Could you check a few things on this model? Use its own coordinates, in mm. A direction names the side the tool comes from. Round coordinates to 2 decimals unless told otherwise and drop trailing zeros. Order: outer loops, then holes, each group sorted by start corner. A loop starts at its lowest first (then second) coordinate and runs counter-clockwise, first axis right, second up.
```python
from build123d import *

# Parameters (mm, degrees)
SKETCH1_W           = 190
SKETCH1_H           = 80
SKETCH1_R           = 1.55
BOSS_EXTRUDE1_DEPTH = 2
SKETCH2_R           = 3
SKETCH2_R_2         = 1.55
BOSS_EXTRUDE2_DEPTH = 12


with BuildPart() as part:
    # Sketch1 → Boss-Extrude1 (new body)
    with BuildSketch(Plane(origin=(0, 0, 0), x_dir=(1, 0, 0), z_dir=(0, 1, 0))):
        with Locations((19.251207729, 0.579710145)):
            Rectangle(SKETCH1_W, SKETCH1_H)
        with Locations(Location((-72.748792271, 37.579710145, 0), (0, 0, 270))):
            Circle(SKETCH1_R, mode=Mode.SUBTRACT)
        with Locations(Location((111.435917928, 37.579710145, 0), (0, 0, 270))):
            Circle(SKETCH1_R, mode=Mode.SUBTRACT)
        with Locations(Location((111.435917928, -36.420289855, 0), (0, 0, 270))):
            Circle(SKETCH1_R, mode=Mode.SUBTRACT)
        with Locations(Location((-72.748792271, -36.420289855, 0), (0, 0, 270))):
            Circle(SKETCH1_R, mode=Mode.SUBTRACT)
    extrude(amount=BOSS_EXTRUDE1_DEPTH)

    # Sketch2 → Boss-Extrude2 (add)
    # profile 1 of 5: a face of its own
    with BuildSketch(Plane(origin=(0, 2, 0), x_dir=(1, 0, 0), z_dir=(0, 1, 0))):
        with Locations(Location((82.711207729, 24.709710145, 0), (0, 0, 270))):
            Circle(SKETCH2_R)
        with Locations(Location((82.711207729, 24.709710145, 0), (0, 0, 270))):
            Circle(SKETCH2_R_2, mode=Mode.SUBTRACT)
    # profile 2 of 5: a face of its own
    with BuildSketch(Plane(origin=(0, 2, 0), x_dir=(1, 0, 0), z_dir=(0, 1, 0))):
        with Locations(Location((80.711207729, -23.550289855, 0), (0, 0, 270))):
            Circle(SKETCH2_R)
        with Locations(Location((80.711207729, -23.550289855, 0), (0, 0, 270))):
            Circle(SKETCH2_R_2, mode=Mode.SUBTRACT)
    # profile 3 of 5: a face of its own
    with BuildSketch(Plane(origin=(0, 2, 0), x_dir=(1, 0, 0), z_dir=(0, 1, 0))):
        with Locations(Location((30.141207729, -8.310289855, 0), (0, 0, 270))):
            Circle(SKETCH2_R)
        with Locations(Location((30.141207729, -8.310289855, 0), (0, 0, 270))):
            Circle(SKETCH2_R_2, mode=Mode.SUBTRACT)
    # profile 4 of 5: a face of its own
    with BuildSketch(Plane(origin=(0, 2, 0), x_dir=(1, 0, 0), z_dir=(0, 1, 0))):
        with Locations(Location((-67.258792271, 33.649710145, 0), (0, 0, 270))):
            Circle(SKETCH2_R)
        with Locations(Location((-67.258792271, 33.649710145, 0), (0, 0, 270))):
            Circle(SKETCH2_R_2, mode=Mode.SUBTRACT)
    # profile 5 of 5: a face of its own
    with BuildSketch(Plane(origin=(0, 2, 0), x_dir=(1, 0, 0), z_dir=(0, 1, 0))):
        with Locations(Location((-67.748792271, -31.930289855, 0), (0, 0, 270))):
            Circle(SKETCH2_R)
        with Locations(Location((-67.748792271, -31.930289855, 0), (0, 0, 270))):
            Circle(SKETCH2_R_2, mode=Mode.SUBTRACT)
    extrude(amount=BOSS_EXTRUDE2_DEPTH)


solid = part.part
```
Q1. Imagine slicing it at B-B, the plane x = 50.5. Please give me the cut outline in (y, z), then the cut area to 3 significant figures.
Q2. For P1, Ø2.5, axis at x = -67.26, z = -33.65, coming from the +Y side; P2, Ø3.5, axis at x = -67.5, z = 32.5, coming from the +Y side; P3, Ø8, axis at x = 19.5, y = 7.5, coming from the -Z side, each with a flat end and sliding along its axis, tell me the tip position at first contact or that it passes through.
Q3. We'd pull the mould along Z, two halves only. Please class faces 1 (the cylindrical face through (27.213, 7.916, 7.66)), 2 (the cylindrical face through (29.548, 7.916, 9.742)), 3 (the flat face through (79, 14, 25)): released by +Z, released by -Z, zero draft, split by the parting line, or undercut.
Q4. Imagine slicing it at C-C, the plane z = -18. Please give me the cut outline in (x, y), then the cut area to 3 significant figures.
Q5. For faces 4 (the flat face through (-67, 2, -34)), 5 (the cylindrical face through (-72.68, 0.99, -39.13)), which set-ups out of +Z, -Z, +X, -X, +Y, -Y let a thin tool reach every point of the face, with its end or its side?
Q6. I need wall thicknesses on L1, parallel to Y at x = 93, z = 33; L2, parallel to X at y = 4, z = 23.5; L3, parallel to X at y = 6, z = 24.5. Which ranges of each line are inside material? Lowest first, please.
Q7. Imagine slicing it at A-A, the plane y = 6.25. State how many separate pieces and enclosed holes the cut face has, then the cut area to 3 significant figures.
Filled in:
1. outline: (0, -40.58) - (2, -40.58) - (2, 39.42) - (0, 39.42) - close
1. area: 160 mm2
2. P1: stops at y = 2
2. P2: stops at y = 14
2. P3: passes through
3. face 1: split by the parting line
3. face 2: undercut
3. face 3: zero draft
4. outline: (-75.75, 0) - (114.25, 0) - (114.25, 2) - (-75.75, 2) - close
4. area: 380 mm2
5. face 4: +Y
5. face 5: +Y, -Y
6. L1: y = 0 to 2
6. L2: x = 77.71 to 79.16, 82.26 to 83.71
6. L3: x = 77.87 to 79.49, 81.94 to 83.56
7. separate pieces: 5
7. enclosed holes: 5
7. area: 104 mm2
